Geometry: final body of the model. Coordinates: model frame, mm. Face numbers are marked on the shaded views. Give positions to 0.01 mm unless a question says otherwise; leave off trailing zeros. Write each loop counter-clockwise with the first axis right and the second up, starting at its lowest first coordinate (ties: lowest second). Pieces come first, ordered by that corner, then holes. Notation, with made-up numbers: (62, 43.5) -> (116, 43.5) arc R28 cw to (116, 63.5) -> close; hole circle Ø6 at (79, -35). An arc over 180 degrees is marked (long way). Answer in a Markdown table with one row per item. Add a question column.
from build123d import *

# Parameters (mm, degrees)
SKETCH2_W           = 101.6
SKETCH2_H           = 300
BOSS_EXTRUDE1_DEPTH = 25.4
SKETCH3_R           = 5.25
SKETCH3_R_2         = 28.575
CUT_EXTRUDE1_DEPTH  = 25.4
SKETCH4_R           = 5.25
CUT_EXTRUDE2_DEPTH  = 25.4


with BuildPart() as part:
    # Sketch2 → Boss-Extrude1 (new body)
    with BuildSketch(Plane(origin=(0, 0, 0), x_dir=(1, 0, 0), z_dir=(0, 1, 0))):
        with Locations((50.8, 150)):
            Rectangle(SKETCH2_W, SKETCH2_H)
    extrude(amount=BOSS_EXTRUDE1_DEPTH)

    # Sketch3 → Cut-Extrude1 (cut)
    with BuildSketch(Plane(origin=(0, 25.4, 0), x_dir=(1, 0, 0), z_dir=(0, 1, 0))):
        with Locations(Location((70.8, 275, 0), (0, 0, 270))):
            Circle(SKETCH3_R)
        with Locations(Location((30.8, 275, 0), (0, 0, 270))):
            Circle(SKETCH3_R)
        with Locations(Location((70.8, 175, 0), (0, 0, 270))):
            Circle(SKETCH3_R)
        with Locations(Location((30.8, 175, 0), (0, 0, 270))):
            Circle(SKETCH3_R)
        with Locations(Location((50.8, 225, 0), (0, 0, 270))):
            Circle(SKETCH3_R_2)
    extrude(amount=-CUT_EXTRUDE1_DEPTH, mode=Mode.SUBTRACT)

    # Sketch4 → Cut-Extrude2 (cut)
    with BuildSketch(Plane(origin=(0, 25.4, 0), x_dir=(1, 0, 0), z_dir=(0, 1, 0))):
        with Locations(Location((70.8, 125, 0), (0, 0, 270))):
            Circle(SKETCH4_R)
        with Locations(Location((30.8, 125, 0), (0, 0, 270))):
            Circle(SKETCH4_R)
        with Locations(Location((30.8, 25, 0), (0, 0, 270))):
            Circle(SKETCH4_R)
        with Locations(Location((70.8, 25, 0), (0, 0, 270))):
            Circle(SKETCH4_R)
    extrude(amount=-CUT_EXTRUDE2_DEPTH, mode=Mode.SUBTRACT)


solid = part.part
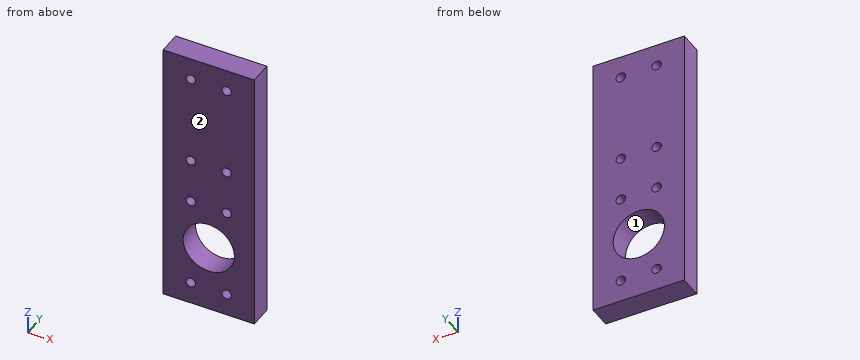
Q1. Pull-direction query (X, two-part tool) for the marked faces 1 and 2; classes: +X half, -X half, draft (parallel to the pull), parting line (faces both ways), or undercut.
Q2. Section B-B on z = -125. Return loops of the section in (x, y).
Q3. Section C-C on x = 50.8. Return loops of the section in (y, z) (3 decimals), and give its area (3 significant figures).
Q4. Section D-D on z = -234. Return loops of the section in (x, y), and give its area (3 significant figures).
Q5. Line query: probe 1 along Z at (x, y) = (52, 6.5); probe 2 along X at (y, z) = (20.25, -125); probe 3 along X at (y, z) = (14.25, -225) (3 decimals). Output: solid intervals per line, ascending. Write a range as from..to.
Q6. Section A-A on y = 13.5. Count the separate pieces of the cut face and the enclosed holes in it, and give its area (3 significant figures).
Q7. Contact query for flat-ended pins moving along their axis: pin 1 Ø17 at (x, z) = (30.8, -25) entering from +Y; pin 2 Ø6.5 at (x, z) = (30.8, -125) entering from -Y. Output: stop coordinate, or through.
Checks:
| question | item | result |
|---|---|---|
| 1 | face 1 | undercut |
| 1 | face 2 | draft |
| 2 | outline | (0, 0) -> (25.55, 0) -> (25.55, 25.4) -> (0, 25.4) -> close; (36.05, 0) -> (65.55, 0) -> (65.55, 25.4) -> (36.05, 25.4) -> close; (76.05, 0) -> (101.6, 0) -> (101.6, 25.4) -> (76.05, 25.4) -> close |
| 3 | outline | (0, -300) -> (25.4, -300) -> (25.4, -253.575) -> (0, -253.575) -> close; (0, -196.425) -> (25.4, -196.425) -> (25.4, 0) -> (0, 0) -> close |
| 3 | area | 6,170 mm^2 |
| 4 | outline | (0, 0) -> (23.68, 0) -> (23.68, 25.4) -> (0, 25.4) -> close; (77.92, 0) -> (101.6, 0) -> (101.6, 25.4) -> (77.92, 25.4) -> close |
| 4 | area | 1,200 mm^2 |
| 5 | probe 1 | -300..-253.55, -196.45..0 |
| 5 | probe 2 | 0..25.55, 36.05..65.55, 76.05..101.6 |
| 5 | probe 3 | 0..22.225, 79.375..101.6 |
| 6 | separate pieces | 1 |
| 6 | enclosed holes | 9 |
| 6 | area | 27,200 mm^2 |
| 7 | pin 1 | y = 25.4 |
| 7 | pin 2 | through |
